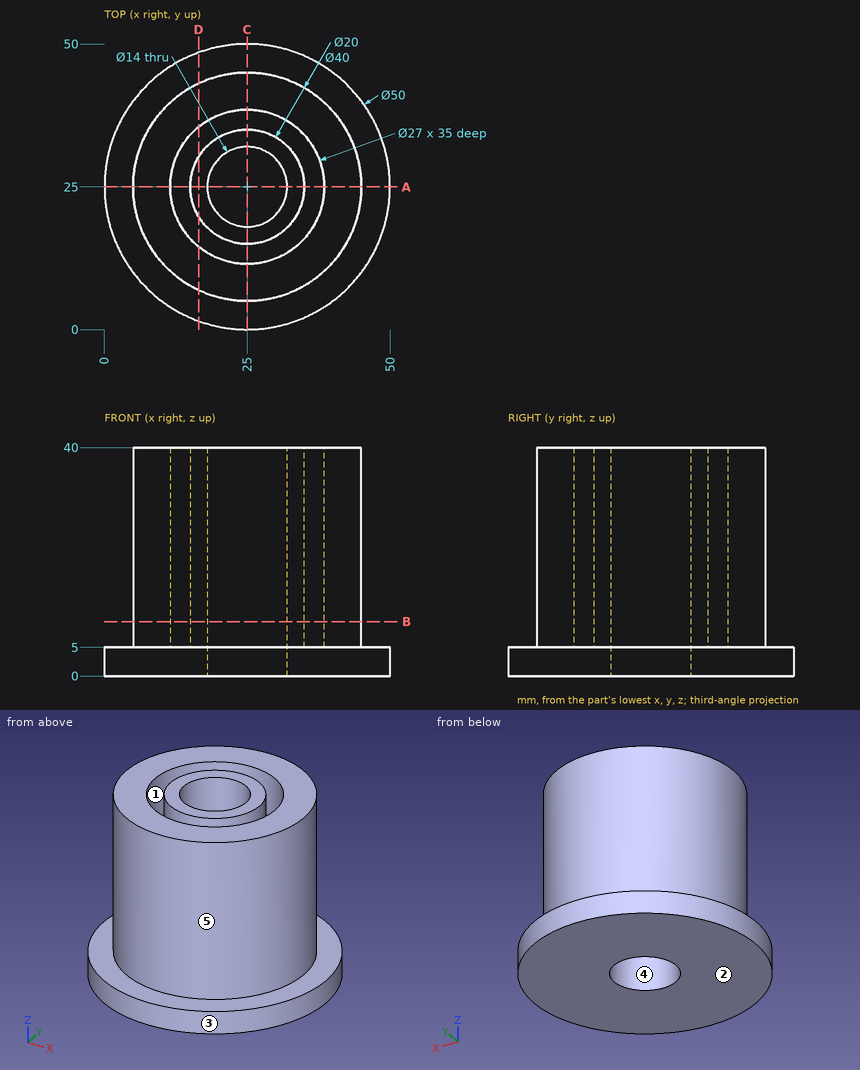
Study the drawing (mm; zero at the part's minimum x, y, z) and answer. A direction names the side the tool comes from. Give positions to 0.01 mm unless a question says otherwise; leave off trailing zeros. Loops run counter-clockwise (first coordinate to the right, second up) from the corner with the lowest first, then second, coordinate; pieces in that order, holes last. Notation, with made-up numbers: (7.5, 87) - (38.5, 87) arc R14 ccw to (38.5, 101) - close; hole circle Ø9 at (-3, 18). An arc over 180 degrees is marked (long way). Return JSON: item names as keys, results as strings. Group by question number.
1. Given pin 1 Ø10 at (x, z) = (12, 14) entering from -Y; pin 2 Ø12 at (y, z) = (42.5, 27.5) entering from -X; pin 3 Ø1.5 at (x, z) = (13.5, 30) entering from -Y; pin 4 Ø11 at (x, y) = (25, 25) entering from -Z (1 decimal), each flat-ended and moving along its own axis, determine where each tip first touches the part or whether it passes through.
2. Which of the six approach directions +Z, -Z, +X, -X, +Y, -Y give full straight-line access (tool end or side, diameter ignored) to the marked faces 4 and 5?
3. Find section B-B (z = 9.5). Write down the section's boundary in (x, y), then the cut area to 3 significant figures.
4. Find section A-A (y = 25). Write down the section's boundary in (x, z), then the cut area to 3 significant figures.
5. Find section D-D (x = 16.5). Write down the section's boundary in (y, z).
6. Determine the mould class of the marked faces 1, 2 and 3 for opening direction Y: pulls with the +Y half, pulls with the -Y half, needs draft (parallel to the pull), parting line crosses it, or undercut.
7. Straight lines are drawn through the part: line 1 (Y direction, x = 25, z = 32); line 2 (X direction, y = 24, z = 6); line 3 (Y direction, x = 22, z = 7.5). For each, find the intervals that lie inside material, in ascending order. Write a range as [from, to].
Verdict:
{
 "1": {"pin 1": "stops at y = 6.67", "pin 2": "stops at x = 8.64", "pin 3": "stops at y = 8.13", "pin 4": "passes through"},
 "2": {"face 4": "+Z, -Z", "face 5": "+Z"},
 "3": {"outline": "circle Ø40 at (25, 25); circle Ø20 at (25, 25); hole circle Ø27 at (25, 25); hole circle Ø14 at (25, 25)", "area": "844 mm^2"},
 "4": {"outline": "(0, 0) - (18, 0) - (18, 40) - (15, 40) - (15, 5) - (11.5, 5) - (11.5, 40) - (5, 40) - (5, 5) - (0, 5) - close; (32, 0) - (50, 0) - (50, 5) - (45, 5) - (45, 40) - (38.5, 40) - (38.5, 5) - (35, 5) - (35, 40) - (32, 40) - close", "area": "845 mm^2"},
 "5": {"outline": "(1.49, 0) - (48.51, 0) - (48.51, 5) - (43.1, 5) - (43.1, 40) - (35.49, 40) - (35.49, 5) - (30.27, 5) - (30.27, 40) - (19.73, 40) - (19.73, 5) - (14.51, 5) - (14.51, 40) - (6.9, 40) - (6.9, 5) - (1.49, 5) - close"},
 "6": {"face 1": "undercut", "face 2": "needs draft", "face 3": "parting line crosses it"},
 "7": {"line 1": "y = [5, 11.5], [15, 18], [32, 35], [38.5, 45]", "line 2": "x = [5.03, 11.54], [15.05, 18.07], [31.93, 34.95], [38.46, 44.97]", "line 3": "y = [5.23, 11.84], [15.46, 18.68], [31.32, 34.54], [38.16, 44.77]"}
}
